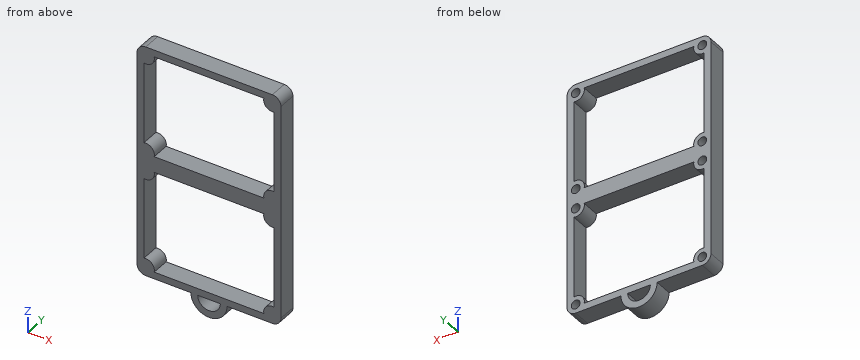
Autodesk Inventor part; units mm, degrees
ref_plane "YZ Plane" through (0, 0, 0) normal (1, 0, 0) x (0, 1, 0)
ref_plane "XZ Plane" through (0, 0, 0) normal (0, 1, 0) x (-1, 0, 0)
ref_plane "XY Plane" through (0, 0, 0) normal (0, 0, 1) x (1, 0, 0)
sketch "Sketch1" plane through (0, 0, 0) normal (0, 1, 0) x (-1, 0, 0)
  circle A0 centre (27.94, -21.59) radius 1.94 construction
  line L0 (3.8945, 0) -> (-7.0745, 0) construction
  line L1 (0, -4.534) -> (0, 5.5912) construction
  circle A1 centre (-27.94, -21.59) radius 1.94 construction
  circle A2 centre (27.94, 21.59) radius 1.94 construction
  circle A3 centre (-27.94, 21.59) radius 1.94 construction
  line L2 (27.94, -25.4) -> (-27.94, -25.4)
  line L3 (31.75, 25.9) -> (-31.75, 25.9) construction
  line L4 (31.75, -21.59) -> (31.75, 25.9)
  line L5 (-31.75, -21.59) -> (-31.75, 25.9)
  line L6 (24.2171, -22.4) -> (-24.2171, -22.4)
  line L7 (24.2171, 22.4) -> (-24.2171, 22.4)
  line L8 (28.75, -17.8671) -> (28.75, 17.8671)
  line L9 (-28.75, -17.8671) -> (-28.75, 17.8671)
  arc A4 (-24.2171, -22.4) -> (-28.75, -17.8671) centre (-27.94, -21.59) ccw
  arc A5 (-31.75, -21.59) -> (-27.94, -25.4) centre (-27.94, -21.59) ccw
  arc A6 (27.94, -25.4) -> (31.75, -21.59) centre (27.94, -21.59) ccw
  arc A7 (28.75, -17.8671) -> (24.2171, -22.4) centre (27.94, -21.59) ccw
  arc A8 (-28.75, 17.8671) -> (-24.2171, 22.4) centre (-27.94, 21.59) ccw
  arc A9 (24.2171, 22.4) -> (28.75, 17.8671) centre (27.94, 21.59) ccw
  circle A10 centre (27.94, 73.39) radius 1.94 construction
  circle A11 centre (-27.94, 73.39) radius 1.94 construction
  circle A12 centre (27.94, 30.21) radius 1.94 construction
  circle A13 centre (-27.94, 30.21) radius 1.94 construction
  line L10 (27.94, 77.2) -> (-27.94, 77.2)
  line L11 (31.75, 73.39) -> (31.75, 25.9)
  line L12 (-31.75, 73.39) -> (-31.75, 25.9)
  line L13 (24.2171, 74.2) -> (-24.2171, 74.2)
  line L14 (24.2171, 29.4) -> (-24.2171, 29.4)
  line L15 (28.75, 69.6671) -> (28.75, 33.9329)
  line L16 (-28.75, 69.6671) -> (-28.75, 33.9329)
  arc A14 (-28.75, 69.6671) -> (-24.2171, 74.2) centre (-27.94, 73.39) ccw
  arc A15 (-27.94, 77.2) -> (-31.75, 73.39) centre (-27.94, 73.39) ccw
  arc A16 (31.75, 73.39) -> (27.94, 77.2) centre (27.94, 73.39) ccw
  arc A17 (24.2171, 74.2) -> (28.75, 69.6671) centre (27.94, 73.39) ccw
  arc A18 (-24.2171, 29.4) -> (-28.75, 33.9329) centre (-27.94, 30.21) ccw
  arc A19 (28.75, 33.9329) -> (24.2171, 29.4) centre (27.94, 30.21) ccw
  arc A20 (-8, -25.4) -> (8, -25.4) centre (0, -25.4) ccw
  arc A21 (-5, -25.4) -> (5, -25.4) centre (0, -25.4) ccw
  point P0 (0, 0)
  dimension "d0" = 3.88
  dimension "d1" = 27.94
  dimension "d2" = 21.59
  dimension "d5" = 55.88
  dimension "d8" = 43.18
  dimension "d11" = 25.4
  dimension "d12" = 31.75
  dimension "d13" = 3
  dimension "d14" = 3
  dimension "d16" = 3.5
  dimension "d17" = 8
  dimension "d18" = 5
extrude "Extrusion1" add sketch "Sketch1" along normal blind 8 contours L2 A5 L5 L12 A15 L10 A16 L11 L4 A6 | A20 L2 A21
sketch "Sketch2" plane through (0, 8, 0) normal (0, 1, 0) x (1, 0, 0)
  line L0 (-31.75, 21.59) -> (-31.75, -73.39)
  line L1 (-8, 25.4) -> (-27.94, 25.4)
  point P0 (0, 0)
  point P1 (-27.94, 21.59)
  dimension "d28" = 3.81
  dimension "d29" = 3.81
hole "Hole1" at (-27.94, 8, -21.59) direction (0, -1, 0) diameter 3.88 depth 5.145 tip angle 118
pattern_linear "Rectangular Pattern1" count 2 spacing 55.88 along (1, 0, 0) count 2 spacing 43.18 along (0, 0, 1) of "Hole1"
pattern_linear "Rectangular Pattern2" count 2 spacing 51.8 along (0, 0, 1) of "Hole1", "Rectangular Pattern1"
properties part number "balloonMount_x2"
Geometry check sheet. Reference: the model listing, model coordinates, mm. Coordinates: 2 decimals unless noted, no trailing zeros. Order: outer loops, then holes, each group sorted by start corner. A loop starts at its lowest first (then second) coordinate and runs counter-clockwise, first axis right, second up. Notation, with made-up numbers: (74, -10.5) - (111, -10.5) arc R26 cw to (111, 7.5) - close; hole circle Ø11 at (25, 75). An arc over 180 degrees is marked (long way). Answer as a JSON object with one key per item and string values. Group by question number.
Item 1: Scan lines: probe 1 along X at (y, z) = (4, 21.59); probe 2 along Z at (x, y) = (15.5, 4.5); probe 3 along X at (y, z) = (2.5, -3). Record each from-to range of solid material in increasing order.
Item 2: Sectioned sample at C-C, the plane y = 4.75. Give the number of separate pieces and of enclosed holes in the cut face, and give its area (3 significant figures).
Item 3: Sectioned sample at A-A, the plane x = 0. Record the cut outline in (y, z), and give its area (3 significant figures).
Item 4: Depth check by flat-ended pin: pin 1 Ø3 at (x, z) = (-27.94, 30.21) entering from -Y; pin 2 Ø2.5 at (x, z) = (-27.94, -21.59) entering from +Y; pin 3 Ø4 at (x, y) = (22, 5.5) entering from -Z; pin 4 Ø4 at (x, y) = (5.5, 2) entering from -Z. Enter the tip coordinate at first touch or a pass-through.
Item 5: Sectioned sample at B-B, the plane x = 12.5. Record the cut outline in (y, z), and give its area (3 significant figures).
Resolved:
{
 "1": {"probe 1": "-31.75 to -29.88, -26 to -24.13, 24.13 to 26, 29.88 to 31.75", "probe 2": "-25.4 to -22.4, 22.4 to 29.4, 74.2 to 77.2", "probe 3": "-31.75 to -28.75, 28.75 to 31.75"},
 "2": {"separate pieces": "1", "enclosed holes": "11", "area": "1,460 mm^2"},
 "3": {"outline": "(0, -33.4) - (8, -33.4) - (8, -30.4) - (0, -30.4) - close; (0, -25.4) - (8, -25.4) - (8, -22.4) - (0, -22.4) - close; (0, 22.4) - (8, 22.4) - (8, 29.4) - (0, 29.4) - close; (0, 74.2) - (8, 74.2) - (8, 77.2) - (0, 77.2) - close", "area": "128 mm^2"},
 "4": {"pin 1": "y = 0", "pin 2": "y = 2.44", "pin 3": "z = -25.4", "pin 4": "z = -32.59"},
 "5": {"outline": "(0, -25.4) - (8, -25.4) - (8, -22.4) - (0, -22.4) - close; (0, 22.4) - (8, 22.4) - (8, 29.4) - (0, 29.4) - close; (0, 74.2) - (8, 74.2) - (8, 77.2) - (0, 77.2) - close", "area": "104 mm^2"}
}
